Input: dimensioned drawing with shaded views. Units: mm. Origin: part minimum x, y, z. Round coordinates to 2 decimals unless told otherwise and drop trailing zeros. Loops run counter-clockwise (first coordinate to the right, second up) from the corner with the lowest first, then second, coordinate; pieces in that order, holes last.
Item 1: Section query D-D on z = 2. Return loops of the section in (x, y), then the cut area to 3 significant figures.
Item 2: Section query A-A on y = 1.65. Give the number of separate pieces and of enclosed holes in the cut face, then the cut area to 3 significant figures.
Item 3: Section query C-C on z = 11.75. Return loops of the section in (x, y).
Item 4: Section query B-B on x = 9. Return loops of the section in (y, z), then the cut area to 3 significant figures.
Item 5: Ray query, L1, parallel to X at y = 1.9, z = 10; L2, parallel to X at y = 1.2, z = 5.75; L3, parallel to Z at x = 53, y = 1.3. Return the intervals inside material, ascending.
Item 6: First-contact query: P1, Ø1, axis at y = 2, z = 17.5, coming from the -X side. Flat tip, straight axial feed; report the tip coordinate or a pass-through.
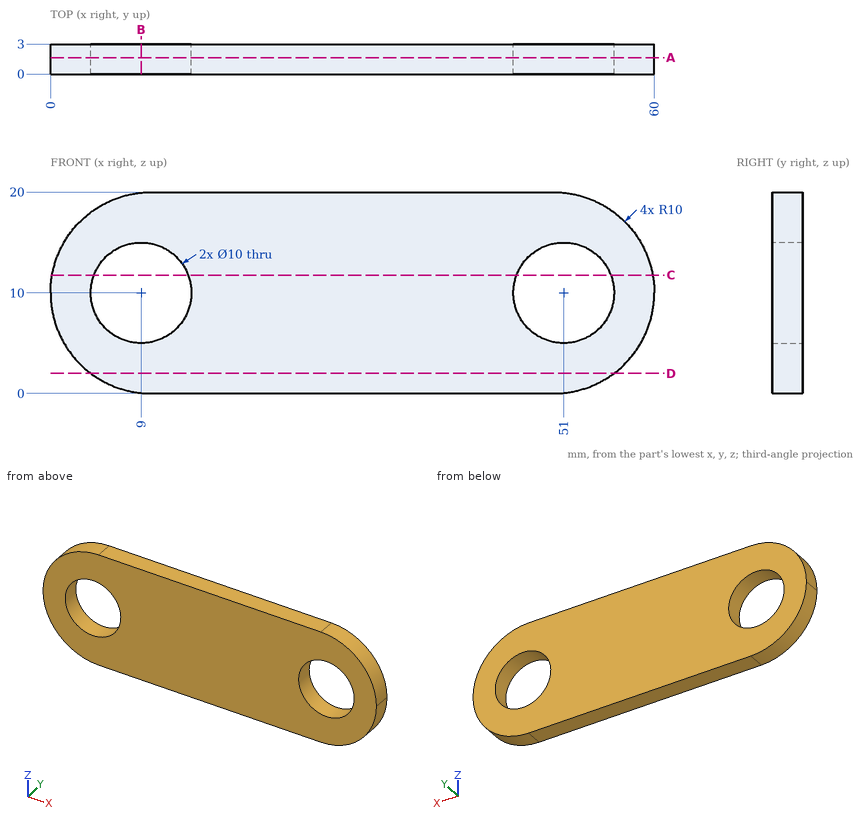
Data:
1. outline: (4, 0) - (56, 0) - (56, 3) - (4, 3) - close
1. area: 156 mm2
2. separate pieces: 1
2. enclosed holes: 2
2. area: 957 mm2
3. outline: (0.15, 0) - (4.32, 0) - (4.32, 3) - (0.15, 3) - close; (13.68, 0) - (46.32, 0) - (46.32, 3) - (13.68, 3) - close; (55.68, 0) - (59.85, 0) - (59.85, 3) - (55.68, 3) - close
4. outline: (0, 0.05) - (3, 0.05) - (3, 5) - (0, 5) - close; (0, 15) - (3, 15) - (3, 19.95) - (0, 19.95) - close
4. area: 29.7 mm2
5. L1: x = 0 to 4, 14 to 46, 56 to 60
5. L2: x = 0.95 to 6.37, 11.63 to 48.37, 53.63 to 59.05
5. L3: z = 0.46 to 5.42, 14.58 to 19.54
6. P1: stops at x = 2.86
